The listing builds one solid part. Answer for the finished solid, in the listing's coordinates (mm). A direction names the side the tool comes from. Coordinates: 2 decimals unless noted, no trailing zeros. Loops run counter-clockwise (first coordinate to the right, second up) from the corner with the lowest first, then second, coordinate; pieces in that order, holes last. Notation, with made-up numbers: M 60,14.5 L 74,14.5 A27 ccw 74,45.5 Z; hole C 31.25,22.5 d11. An arc over 180 degrees is marked long. Return JSON: item names as keys, results as strings. Group by question number.
1. Section B-B (z = 8.75) is taken. Write down the section's boundary in (x, y), then the cut area to 3 significant figures.
2. Straight lines are drawn through the part: L1, parallel to Y at x = 7, z = 4.2; L2, parallel to Z at x = 7.75, y = -1.5; L3, parallel to Y at x = 7.75, z = 2.75. For each, find the intervals that lie inside material, in ascending order. Write a range as from..to.
3. The mould has two halves that part along Z. Classify faces 1 (the face through (12, -22, 20)), 2 (the face through (14, -22, 8)), 3 (the face through (7, -22, 25.5)), 4 (the face through (7, -22, 0)): pulls with the +Z half, pulls with the -Z half, needs draft (parallel to the pull), parting line crosses it, or undercut.
4. Which of the six approach directions +Z, -Z, +X, -X, +Y, -Y give full straight-line access (tool end or side, diameter ignored) to faces 5 (the face through (12.57, -14, 15.64)), 6 (the face through (12.5, -29.07, 15.64)), 7 (the face through (1.5, -29.07, 15.64))?
5. Section A-A (y = -6.25) is taken. Write down the section's boundary in (x, z).
6. Given P1, Ø7, axis at x = 5.5, y = -38, coming from the +Z side; P2, Ø6, axis at x = 11.5, z = 20.5, coming from the -Y side; P3, Ø3.5, axis at y = -23, z = 19.5, coming from the -X side, each flat-ended and moving along its own axis, determine where each tip first touches the part or whether it passes through.
7. Section D-D (y = -21.5) is taken. Write down the section's boundary in (x, z), then the cut area to 3 significant figures.
8. Section C-C (x = 7) is taken. Write down the section's boundary in (y, z) (3 decimals).
```python
from build123d import *

# Parameters (mm, degrees)
F0_W     = 18
F0_H     = 20
F1_DEPTH = 14
F2_R     = 2.5
F3_DEPTH = 5.8
F4_R     = 5
F5_R     = 3.725
F6_DEPTH = 12


with BuildPart() as f1:
    # F0 (on Right) → F1 (new body)
    with BuildSketch(Plane.YZ):
        with Locations((-21.5, 15.5)):
            Rectangle(F0_W, F0_H)
        Polygon((-43, 0), (0, 0), (0, 5.5), (-12.5, 5.5), (-30.5, 5.5), (-43, 5.5), align=None)
    extrude(amount=F1_DEPTH)

    # F2 (on face) → F3 (cut)
    with BuildSketch(Plane.XY.offset(5.5)):
        with Locations((7, -6.25)):
            Circle(F2_R)
        with Locations((7, -36.75)):
            Circle(F2_R)
    extrude(amount=-F3_DEPTH, mode=Mode.SUBTRACT)

    # F4
    f4_edges = [f1.edges().sort_by_distance(p)[0] for p in [
        (7, -30.5, 25.5),
        (7, -12.5, 25.5),
        (14, -30.5, 15.5),
        (14, -12.5, 15.5),
        (0, -12.5, 15.5),
        (0, -30.5, 15.5),
    ]]
    fillet(f4_edges, radius=F4_R)

    # F5 (on face) → F6 (cut)
    with BuildSketch(Plane.YZ):
        with Locations((-21.5, 19.775)):
            Circle(F5_R)
    extrude(amount=F6_DEPTH, mode=Mode.SUBTRACT)


solid = f1.part
```
Worked out:
{
 "1": {"outline": "M 0,-25.5 A5 ccw 5,-30.5 L 9,-30.5 A5 ccw 14,-25.5 L 14,-17.5 A5 ccw 9,-12.5 L 5,-12.5 A5 ccw 0,-17.5 Z", "area": "231 mm^2"},
 "2": {"L1": "-43..-39.25, -34.25..-8.75, -3.75..0", "L2": "0..5.5", "L3": "-43..-39.13, -34.37..-8.63, -3.87..0"},
 "3": {"face 1": "undercut", "face 2": "needs draft", "face 3": "pulls with the +Z half", "face 4": "pulls with the -Z half"},
 "4": {"face 5": "+Z, +X, +Y", "face 6": "+Z, +X, -Y", "face 7": "+Z, -X, -Y"},
 "5": {"outline": "M 0,0 L 4.5,0 L 4.5,5.5 L 0,5.5 Z; M 9.5,0 L 14,0 L 14,5.5 L 9.5,5.5 Z"},
 "6": {"P1": "z = 5.5", "P2": "y = -30.5", "P3": "x = 12"},
 "7": {"outline": "M 0,0 L 14,0 L 14,25.5 L 0,25.5 L 0,23.5 L 12,23.5 L 12,16.05 L 0,16.05 Z", "area": "268 mm^2"},
 "8": {"outline": "M -43,0 L -39.25,0 L -39.25,5.5 L -43,5.5 Z; M -34.25,0 L -8.75,0 L -8.75,5.5 L -12.5,5.5 L -12.5,20.5 A5 ccw -17.5,25.5 L -25.5,25.5 A5 ccw -30.5,20.5 L -30.5,5.5 L -34.25,5.5 Z; M -3.75,0 L 0,0 L 0,5.5 L -3.75,5.5 Z; hole C -21.5,19.775 d7.45"}
}
